Autodesk Inventor part; units mm, degrees
ref_plane "YZ Plane" through (0, 0, 0) normal (1, 0, 0) x (0, 1, 0)
ref_plane "XZ Plane" through (0, 0, 0) normal (0, 1, 0) x (-1, 0, 0)
ref_plane "XY Plane" through (0, 0, 0) normal (0, 0, 1) x (1, 0, 0)
sketch "Sketch1" plane through (0, 0, 0) normal (0, 0, 1) x (1, 0, 0)
  circle A0 centre (0, 0) radius 7.9375
  dimension "d0" = 15.875
extrude "Extrusion1" add sketch "Sketch1" along normal blind 15.875
sketch "Sketch2" plane through (0, 0, 15.875) normal (0, 0, 1) x (1, 0, 0)
  circle A0 centre (0, 0) radius 11.1125
  dimension "d3" = 22.225
extrude "Extrusion2" add sketch "Sketch2" along normal blind 174.625
sketch "Sketch3" plane through (0, 0, 190.5) normal (0, 0, 1) x (1, 0, 0)
  circle A0 centre (0, 0) radius 7.9375
extrude "Extrusion3" add sketch "Sketch3" along normal blind 12.7
sketch "Sketch4" plane through (0, 0, 0) normal (0, 0, -1) x (-1, 0, 0)
  line L0 (-4.7625, 0) -> (4.7625, 0) construction
  line L1 (-4.7625, 14.2513) -> (-13.4248, 14.2513)
  line L2 (-13.4248, 14.2513) -> (-13.4248, -14.2513)
  line L3 (-13.4248, -14.2513) -> (-4.7625, -14.2513)
  line L4 (-4.7625, -14.2513) -> (-4.7625, 14.2513)
  line L5 (4.7625, 14.2513) -> (11.8991, 14.2513)
  line L6 (11.8991, 14.2513) -> (11.8991, -14.2513)
  line L7 (11.8991, -14.2513) -> (4.7625, -14.2513)
  line L8 (4.7625, -14.2513) -> (4.7625, 14.2513)
  point P0 (0, 0)
  point P1 (0, 0)
  dimension "d8" = 9.525
extrude "Extrusion4" cut sketch "Sketch4" against normal up to surface (15.875 mm away)
sketch "Sketch5" plane through (4.7625, -6.35, 0) normal (1, 0, 0) x (0, 0, -1)
  line L0 (0, 6.35) -> (-6.35, 6.35) construction
  circle A0 centre (-6.35, 6.35) radius 3.175
  dimension "d11" = 6.35
  dimension "d12" = 6.35
extrude "Extrusion5" cut sketch "Sketch5" against normal through all
sketch "Sketch6" plane through (0, 0, 203.2) normal (0, 0, 1) x (1, 0, 0)
  line L0 (-6.35, 6.35) -> (6.35, 6.35)
  line L1 (6.35, 6.35) -> (6.35, -6.35)
  line L2 (6.35, -6.35) -> (-6.35, -6.35)
  line L3 (-6.35, -6.35) -> (-6.35, 6.35)
  line L4 (0, 0) -> (0, 6.35) construction
  line L5 (0, 0) -> (-6.35, 0) construction
  dimension "d15" = 12.7
extrude "Extrusion6" add sketch "Sketch6" along normal blind 28.575
sketch "Sketch7" plane through (0, 0, 231.775) normal (0, 0, 1) x (1, 0, 0)
  line L0 (-4.7625, 6.35) -> (4.7625, 6.35)
  line L1 (4.7625, -6.35) -> (-4.7625, -6.35)
  line L2 (-3.175, 6.35) -> (3.175, 6.35)
  line L3 (3.175, 6.35) -> (3.175, -6.35)
  line L4 (3.175, -6.35) -> (-3.175, -6.35)
  line L5 (-3.175, -6.35) -> (-3.175, 6.35)
  line L6 (-3.175, 0) -> (3.175, 0) construction
  point P0 (0, 0)
  point P1 (0, 0)
  dimension "d18" = 6.35
extrude "Extrusion7" cut sketch "Sketch7" against normal blind 15.875
sketch "Sketch8" plane through (6.35, 4.7625, 203.2) normal (1, 0, 0) x (0, 0, -1)
  line L0 (-28.575, -11.1125) -> (-28.575, 1.5875) construction
  line L1 (-28.575, -4.7625) -> (-22.225, -4.7625) construction
  circle A0 centre (-22.225, -4.7625) radius 3.175
  point P0 (203.2, -4.7625)
  dimension "d21" = 6.35
  dimension "d22" = 6.35
extrude "Extrusion8" cut sketch "Sketch8" against normal through all
thread "Thread1"
thread "Thread2"
thread "Thread3"
properties part number "4in stroke cylinder"
Source: CAD feature listing. Evaluate the final solid. Frame: model axes, mm. A direction names the side the tool comes from. Give positions to 0.01 mm unless a question says otherwise; leave off trailing zeros. Use a Markdown table: item, result.
1) Reachability of faces 1 (the cylindrical face through (-0.072, 7.937, 7.826)), 2 (the cylindrical face through (0.072, -7.937, 7.826)), 3 (the flat face through (0, 0, 215.9)), 4 (the flat face through (0, 6.35, 214)), 5 (the flat face through (6.35, 0, 217)) from +Z, -Z, +X, -X, +Y, -Y: full face, straight path, thin tool, end or side. Return the list, or none.
Answer list:
| item | result |
|---|---|
| face 1 | -Z, +Y |
| face 2 | -Z, -Y |
| face 3 | +Z, +Y, -Y |
| face 4 | +Z, +X, -X, +Y |
| face 5 | +Z, +X, +Y, -Y |
2) Mould query, pull axis X, two halves, no side actions, for faces 6 (the flat face through (-3.175, 0, 222)), 7 (the cylindrical face through (-4.74, -1.216, 222.492)), 8 (the flat face through (-6.35, 0, 217)). Classes: +X half, -X half, draft (parallel to the pull), parting line (faces both ways), or undercut.
Answer list:
| item | result |
|---|---|
| face 6 | undercut |
| face 7 | draft |
| face 8 | -X half |
3) Contact query for flat-ended pins moving along their axis: P1, Ø1.9, axis at x = -1.5, y = 1.5, coming from the +Z side; P2, Ø2, axis at y = 2, z = 203.5, coming from the +X side; P3, Ø0.8, axis at x = -7.5, y = 2, coming from the +Z side; P4, Ø5, axis at y = 0, z = 225.425, coming from the -X side. Output: stop coordinate, or through.
Answer list:
| item | result |
|---|---|
| P1 | z = 215.9 |
| P2 | x = 7.87 |
| P3 | z = 203.2 |
| P4 | through |
4) Section query C-C, the plane y = 0. Count the separate pieces of the cut face and the enclosed holes in it, then the cut area to 3 significant figures.
Answer list:
| item | result |
|---|---|
| separate pieces | 4 |
| enclosed holes | 0 |
| area | 4,400 mm² |
5) Ray query, line 1 along X through (y, z) = (2, 216) (3 decimals); line 2 along Y through (x, z) = (-1, 6.35) (3 decimals); line 3 along Z through (x, y) = (4.25, 0.75) (3 decimals). Return the intervals inside material, ascending. Write a range as [from, to].
Answer list:
| item | result |
|---|---|
| line 1 | [-6.35, -3.175], [3.175, 6.35] |
| line 2 | [-7.874, -3.175], [3.175, 7.874] |
| line 3 | [0, 3.265], [9.435, 222.34], [228.51, 231.775] |
